Design review of the part shown in the three views and the two pictorial views. Dimensions are in mm from the part's minimum x, y and z. A direction names the side the tool comes from. Round coordinates to 2 decimals unless told otherwise and drop trailing zeros. Order: outer loops, then holes, each group sorted by start corner. A loop starts at its lowest first (then second) coordinate and runs counter-clockwise, first axis right, second up.
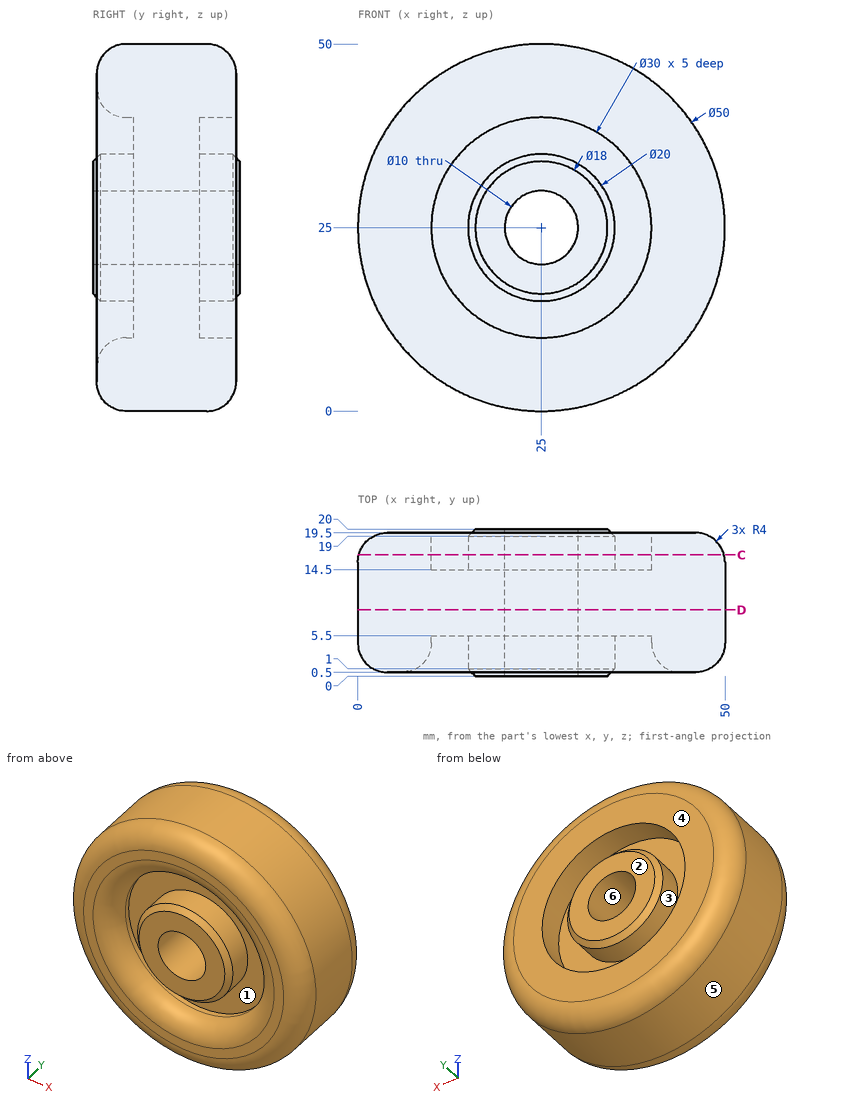
(1) Add section C-C on y = 16.5. Give the boundary of the cut face in (x, z), plus the area to 3 significant figures.
(2) Add section D-D on y = 9. Give the boundary of the cut face in (x, z).
(3) Clearance check with flat-ended pins moving along their axes: P1, Ø18, axis at x = 25, z = 25, coming from the +Y side; P2, Ø2, axis at x = 20, y = 10, coming from the -Z side; P3, Ø4, axis at x = 13, y = 8, coming from the -Z side; P4, Ø3, axis at x = 35, y = 14, coming from the -Z side. State where each tip first meets the part, or that it passes through.
(4) Tool access review of the marked faces 1, 2 and 3: name each direction out of +Z, -Z, +X, -X, +Y, -Y from which nothing blocks a thin tool from reaching the whole face with its end or side.
(5) Wall thickness on L1, parallel to X at y = 4.8, z = 25; L2, parallel to X at y = 17.05, z = 25; L3, parallel to X at y = 10.25, z = 25: over which ranges is each line inside the solid? List them lowest first.
(6) Draft analysis for pull direction Z (two halves, no side actions). For the marked faces 4, 5 and 6, state which applies: pulls with the +Z half, pulls with the -Z half, needs draft (parallel to the pull), parting line crosses it, or undercut.
Here are the results:
1. outline: circle Ø49.75 at (25, 25); circle Ø20 at (25, 25); hole circle Ø30 at (25, 25); hole circle Ø10 at (25, 25)
1. area: 1,470 mm2
2. outline: circle Ø50 at (25, 25); hole circle Ø10 at (25, 25)
3. P1: stops at y = 20
3. P2: stops at z = 0.32
3. P3: stops at z = 2.09
3. P4: stops at z = 1.49
4. face 1: -Y
4. face 2: +Z, -Z, +X, -X, +Y
4. face 3: +Y
5. L1: x = 0 to 10, 15 to 20, 30 to 35, 40 to 50
5. L2: x = 0.31 to 10, 15 to 20, 30 to 35, 40 to 49.69
5. L3: x = 0 to 20, 30 to 50
6. face 4: needs draft
6. face 5: parting line crosses it
6. face 6: undercut
